Geometry check sheet. Reference: the model listing, model coordinates, mm. A direction names the side the tool comes from. Coordinates: 2 decimals unless noted, no trailing zeros. Write each loop counter-clockwise with the first axis right and the second up, starting at its lowest first coordinate (ties: lowest second). Pieces come first, ordered by that corner, then holes. Notation, with made-up numbers: (79.25, -16.5) -> (123.25, -16.5) arc R20 cw to (123.25, 18.5) -> close; hole circle Ø6 at (73, 7.5). An arc over 180 degrees is marked (long way). Answer in a Markdown table with one row per item. Add a question column.
Q1. Gauge pin test, flat ends, axial feed: P1, Ø2, axis at x = 3, y = -1.5, coming from the -Z side; P2, Ø1.1, axis at x = 0.5, y = -1, coming from the -Z side; P3, Ø1, axis at x = 4.5, y = -2, coming from the -Z side. Record the tip position at first contact, or that the pin passes through.
Q2. Section check B-B, the plane x = 4. Record the boundary of the cut face in (y, z).
Q3. Section check D-D, the plane y = -1.05. Record the boundary of the cut face in (x, z), and give its area (3 significant figures).
Q4. Section check A-A, the plane y = 0. Record the boundary of the cut face in (x, z).
Q5. Thickness scan on line 1 (Z direction, x = 4, y = 0); line 2 (X direction, y = 0.7, z = -0.75). Record the ranges inside material, lowest first.
Q6. Tool access check on faces 1 (the face through (6.5, 1, -1)), 2 (the face through (2, 0, 0)), 3 (the face through (0.5, 0, -0.5)). Record the directions out of +Z, -Z, +X, -X, +Y, -Y that give a thin tool (end or side, any length) a straight path to the whole face; none if there is none.
Q7. Release check for a two-part mould opening along Z. For faces 4 (the face through (0, 0, 1)), 5 (the face through (4.22, -0.27, 1.22)), 6 (the face through (3.296, 2.385, -0.751)) record: pulls with the +Z half, pulls with the -Z half, needs draft (parallel to the pull), parting line crosses it, or undercut.
Q8. Section check C-C, the plane z = 0. Record the boundary of the cut face in (x, y).
```python
from build123d import *

# Parameters (mm, degrees)
SKETCH2_W          = 1
SKETCH2_H          = 5
CUT_EXTRUDE1_DEPTH = 1


with BuildPart() as part:
    # Sketch1 → Revolve1 (revolve)
    with BuildSketch(Plane.XY):
        Polygon((0, 0), (0, 2.5), (6.5, 2.5), (6.5, 1.25), (2, 1.25), (2, 0), align=None)
    revolve(axis=Axis((2, 0, 0), (-1, 0, 0)))

    # Sketch2 → Cut-Extrude1 (cut)
    with BuildSketch(Plane.ZY):
        Rectangle(SKETCH2_W, SKETCH2_H)
    extrude(amount=-CUT_EXTRUDE1_DEPTH, mode=Mode.SUBTRACT)


solid = part.part
```
Calculated:
| question | item | result |
|---|---|---|
| 1 | P1 | stops at z = -2.45 |
| 1 | P2 | stops at z = -2.46 |
| 1 | P3 | stops at z = -2 |
| 2 | outline | circle Ø5 at (0, 0); hole circle Ø2.5 at (0, 0) |
| 3 | outline | (0, -2.27) -> (6.5, -2.27) -> (6.5, -0.68) -> (2, -0.68) -> (2, 0.68) -> (6.5, 0.68) -> (6.5, 2.27) -> (0, 2.27) -> (0, 0.5) -> (1, 0.5) -> (1, -0.5) -> (0, -0.5) -> close |
| 3 | area | 22.4 mm² |
| 4 | outline | (0, -2.5) -> (6.5, -2.5) -> (6.5, -1.25) -> (2, -1.25) -> (2, 1.25) -> (6.5, 1.25) -> (6.5, 2.5) -> (0, 2.5) -> (0, 0.5) -> (1, 0.5) -> (1, -0.5) -> (0, -0.5) -> close |
| 5 | line 1 | z = -2.5 to -1.25, 1.25 to 2.5 |
| 5 | line 2 | x = 0 to 2 |
| 6 | face 1 | +Z, -Z, +X, +Y, -Y |
| 6 | face 2 | +X |
| 6 | face 3 | -X, +Y, -Y |
| 7 | face 4 | needs draft |
| 7 | face 5 | undercut |
| 7 | face 6 | parting line crosses it |
| 8 | outline | (1, -2.5) -> (6.5, -2.5) -> (6.5, -1.25) -> (2, -1.25) -> (2, 1.25) -> (6.5, 1.25) -> (6.5, 2.5) -> (1, 2.5) -> close |
